Can you work these out from the model? Positions are in its coordinate system, mm. Round coordinates to 2 decimals unless told otherwise and drop trailing zeros. Write each loop counter-clockwise with the first axis right and the second up, starting at its lowest first coordinate (ties: lowest second). Pieces come first, ordered by that corner, then holes. Notation, with made-up numbers: M 68,-10.75 L 88,-10.75 A38 ccw 88,27.25 Z; hole C 27,66.5 d7. An arc over 180 degrees is marked long. Answer as a JSON object with one key per item and string values. Group by question number.
1) Suppose I cut it at D-D, the plane x = 1.55. Write out the boundary of the cut face in (y, z) (3 decimals).
2) Suppose I cut it at C-C, the plane z = 0. Write out the boundary of the cut face in (x, y) (3 decimals).
3) Suppose I cut it at A-A, the plane y = 0. Write out the boundary of the cut face in (x, z) (3 decimals).
4) If we mould it in two halves opening along Z, with no side actions, what happens to faces 1 (the cylindrical face through (1.127, -33.541, 30.818)), 2 (the flat face through (1, 38.1, 1)), 3 (the flat face through (1, -1, 38.1))? For each: +Z half, -Z half, draft (parallel to the pull), parting line (faces both ways), or undercut.
5) Please list where these lines run through material, in increasing order: L1, parallel to Y at x = 1.5, z = 32; L2, parallel to Y at x = 0.65, z = 0 (3 decimals); L3, parallel to Y at x = 1.3, z = 33. Write a range as [from, to].
6) Suppose I cut it at B-B, the plane y = 31.75. Write out the boundary of the cut face in (x, z), and give its area (3 significant figures).
from build123d import *

# Parameters (mm, degrees)
SKETCH1_W           = 76.2
SKETCH1_H           = 76.2
SKETCH1_R           = 2.5527
SKETCH1_R_2         = 2.0193
SKETCH1_R_3         = 9.525
BOSS_EXTRUDE1_DEPTH = 2.286


with BuildPart() as part:
    # Sketch1 → Boss-Extrude1 (new body)
    with BuildSketch(Plane(origin=(0, 0, 0), x_dir=(0, 0, -1), z_dir=(1, 0, 0))):
        Rectangle(SKETCH1_W, SKETCH1_H)
        with Locations((-25.4, 0)):
            Circle(SKETCH1_R, mode=Mode.SUBTRACT)
        with Locations((-31.75, 31.75)):
            Circle(SKETCH1_R_2, mode=Mode.SUBTRACT)
        Circle(SKETCH1_R_3, mode=Mode.SUBTRACT)
        with Locations((25.4, 0)):
            Circle(SKETCH1_R, mode=Mode.SUBTRACT)
        with Locations((31.75, 31.75)):
            Circle(SKETCH1_R_2, mode=Mode.SUBTRACT)
        with Locations((31.75, -31.75)):
            Circle(SKETCH1_R_2, mode=Mode.SUBTRACT)
        with Locations((-31.75, -31.75)):
            Circle(SKETCH1_R_2, mode=Mode.SUBTRACT)
    extrude(amount=BOSS_EXTRUDE1_DEPTH)


solid = part.part
Results:
{
 "1": {"outline": "M -38.1,-38.1 L 38.1,-38.1 L 38.1,38.1 L -38.1,38.1 Z; hole C -31.75,-31.75 d4.039; hole C -31.75,31.75 d4.039; hole C 0,0 d19.05; hole C 0,-25.4 d5.105; hole C 0,25.4 d5.105; hole C 31.75,-31.75 d4.039; hole C 31.75,31.75 d4.039"},
 "2": {"outline": "M 0,-38.1 L 2.286,-38.1 L 2.286,-9.525 L 0,-9.525 Z; M 0,9.525 L 2.286,9.525 L 2.286,38.1 L 0,38.1 Z"},
 "3": {"outline": "M 0,-38.1 L 2.286,-38.1 L 2.286,-27.953 L 0,-27.953 Z; M 0,-22.847 L 2.286,-22.847 L 2.286,-9.525 L 0,-9.525 Z; M 0,9.525 L 2.286,9.525 L 2.286,22.847 L 0,22.847 Z; M 0,27.953 L 2.286,27.953 L 2.286,38.1 L 0,38.1 Z"},
 "4": {"face 1": "undercut", "face 2": "draft", "face 3": "+Z half"},
 "5": {"L1": "[-38.1, -33.75], [-29.75, 29.75], [33.75, 38.1]", "L2": "[-38.1, -9.525], [9.525, 38.1]", "L3": "[-38.1, -33.34], [-30.16, 30.16], [33.34, 38.1]"},
 "6": {"outline": "M 0,-38.1 L 2.29,-38.1 L 2.29,-33.77 L 0,-33.77 Z; M 0,-29.73 L 2.29,-29.73 L 2.29,29.73 L 0,29.73 Z; M 0,33.77 L 2.29,33.77 L 2.29,38.1 L 0,38.1 Z", "area": "156 mm^2"}
}
